from build123d import *
from build123d import SkipClean  # not in build123d's __all__

# Parameters (mm, degrees)
F1_DEPTH = 2
F2_DEPTH = 50
F3_R     = 9.5
F3_R_2   = 7.5
F4_DEPTH = 5
F5_DEPTH = 20
F6_DEPTH = 60
F8_DEPTH = 2


# Not quite as in the source:
# - a feature names something its author has since deleted; it is built from what else it names


with BuildPart() as f1:
    # F0 (on Front) → F1 (new body)
    with BuildSketch(Plane.XZ):
        with BuildLine():
            Line((21.9700236311, 14.0702866067), (21.9700236311, 12.0961134337))
            ThreePointArc((21.9700236311, 12.0961134337), (22.5646192045, 13.0834230481), (23.1148758296, 14.0961134337))
            Line((23.1148758296, 14.0961134337), (23.1148758296, 16.4762131806))
            ThreePointArc((23.1148758296, 16.4762131806), (22.5745245911, 15.2579871773), (21.9700236311, 14.0702866067))
        make_face()
        with BuildLine():
            ThreePointArc((25, 26), (-24.2306684883, 32.1542428138), (21.9700236311, 14.0702866067))
            ThreePointArc((21.9700236311, 14.0702866067), (22.5745245911, 15.2579871773), (23.1148758296, 16.4762131806))
            ThreePointArc((23.1148758296, 16.4762131806), (24.5241910747, 21.1457181654), (25, 26))
        make_face()
    extrude(amount=F1_DEPTH)

    # F0 (on Front) → F2 (join)
    with BuildSketch(Plane.XZ):
        with BuildLine():
            ThreePointArc((23.1148758296, 14.0961134337), (25.2684266583, 19.8757356184), (26, 26))
            ThreePointArc((26, 26), (-24.9721906769, 33.2380724503), (21.9700236311, 12.0961134337))
            Line((21.9700236311, 12.0961134337), (21.9700236311, 14.0702866067))
            ThreePointArc((21.9700236311, 14.0702866067), (-24.2306684883, 32.1542428138), (25, 26))
            ThreePointArc((25, 26), (24.5241910747, 21.1457181654), (23.1148758296, 16.4762131806))
            Line((23.1148758296, 16.4762131806), (23.1148758296, 14.0961134337))
        make_face()
    extrude(amount=F2_DEPTH)

    # F3 (on Top) → F4 (join)
    with BuildSketch(Plane.XY):
        with Locations((0, -25)):
            Circle(F3_R)
        with Locations((0, -25)):
            Circle(F3_R_2, mode=Mode.SUBTRACT)
    with SkipClean():  # cleaning this boolean's faces spoils the solid; the shape is the same uncleaned
        extrude(amount=F4_DEPTH)

    # F3 (on Top) → F5 (join)
    with BuildSketch(Plane.XY):
        with Locations((0, -25)):
            Circle(F3_R)
        with Locations((0, -25)):
            Circle(F3_R_2, mode=Mode.SUBTRACT)
    extrude(amount=-F5_DEPTH)

    # F6 (cut): a face of the model
    f6_faces = [f1.faces().sort_by_distance(p)[0] for p in [
        (0.0283286742, -2, 25.9851504248),
    ]]
    extrude(f6_faces, amount=F6_DEPTH, mode=Mode.SUBTRACT)

    # F7 (on face) → F8 (join)
    with BuildSketch(Plane.XZ.offset(50)):
        Polygon((23.1148758296, 16.4762131806), (21.9700236311, 14.0702866067), (21.9700236311, 12.0961134337), (23.1148758296, 14.0961134337), align=None)
    extrude(amount=-F8_DEPTH)


solid = f1.part
Source: CAD feature listing. Evaluate the final solid. Frame: model axes, mm. Round coordinates to 2 decimals unless told otherwise and drop trailing zeros. Loops run counter-clockwise (first coordinate to the right, second up) from the corner with the lowest first, then second, coordinate; pieces in that order, holes last.
Q1. Section C-C, the plane x = 0. Return loops of the section in (y, z).
Q2. Section D-D, the plane z = -9. Return loops of the section in (x, y).
Q3. First-contact query: P1, Ø1, axis at x = -2, z = 43, coming from the -Y side; P2, Ø2, axis at y = -29.5, z = 33.5, coming from the +X side; P3, Ø4, axis at y = -13.5, z = 17.5, coming from the -X side. Flat tips, straight axial feed; report the tip coordinate or a pass-through.
Q4. Mould query, pull axis X, two halves, no side actions, for faces 1 (the face through (22.55, -49.01, 15.29)), 2 (the face through (21.97, -25, 13)), 3 (the face through (-1.24, -15.58, -9.25)), 4 (the face through (7.154, -22.747, -9.299)). Classes: pulls with the +X half, pulls with the -X half, needs draft (parallel to the pull), parting line crosses it, or undercut.
Q5. Section A-A, the plane y = -25. Return loops of the section in (x, z).
Q6. Ray query, line 1 (Z direction, x = 1, y = -15.5); line 2 (X direction, y = -25, z = -6); line 3 (Y direction, x = 0, z = -8.75). Return the intervals inside material, ascending.
Q7. Section B-B, the plane z = 30.5. Return loops of the section in (x, y), plus the area to 3 significant figures.
Solutions:
1. outline: (-50, 0) - (-34.5, 0) - (-34.5, -20) - (-32.5, -20) - (-32.5, 0) - (-17.5, 0) - (-17.5, -20) - (-15.5, -20) - (-15.5, 0) - (0, 0) - (0, 52) - (-50, 52) - (-50, 51) - (-2, 51) - (-2, 1) - (-50, 1) - close
2. outline: circle Ø19 at (0, -25); hole circle Ø15 at (0, -25)
3. P1: stops at y = -2
3. P2: stops at x = 25.17
3. P3: stops at x = -25.17
4. face 1: undercut
4. face 2: pulls with the +X half
4. face 3: parting line crosses it
4. face 4: undercut
5. outline: (-9.5, -20) - (-7.5, -20) - (-7.5, 1.11) arc R26 ccw to (7.5, 1.11) - (7.5, -20) - (9.5, -20) - (9.5, 1.8) arc R26 ccw to (21.97, 12.1) - (21.97, 14.07) arc R25 cw (long way) to (23.11, 16.48) - (23.11, 14.1) arc R26 ccw (long way) to (-9.5, 1.8) - close
6. line 1: z = 0.02 to 1.02, 50.98 to 51.98
6. line 2: x = -9.5 to -7.5, 7.5 to 9.5
6. line 3: y = -34.5 to -32.5, -17.5 to -15.5
7. outline: (-25.61, -50) - (-24.59, -50) - (-24.59, -2) - (24.59, -2) - (24.59, -50) - (25.61, -50) - (25.61, 0) - (-25.61, 0) - close
7. area: 200 mm2
